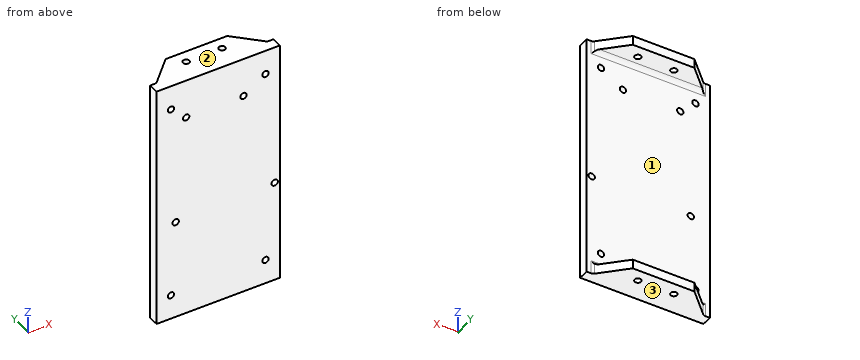
Autodesk Inventor part; units mm, degrees
ref_plane "YZ Plane" through (0, 0, 0) normal (1, 0, 0) x (0, 1, 0)
ref_plane "XZ Plane" through (0, 0, 0) normal (0, 1, 0) x (-1, 0, 0)
ref_plane "XY Plane" through (0, 0, 0) normal (0, 0, 1) x (1, 0, 0)
sketch "Sketch1" plane through (0, 0, 0) normal (0, 1, 0) x (-1, 0, 0)
  line L0 (0, 0) -> (60, 0)
  line L1 (60, 0) -> (60, -120)
  line L2 (60, -120) -> (0, -120)
  line L3 (0, -120) -> (0, 0)
  dimension "d0" = 60
  dimension "d1" = 120
extrude "Extrusion1" add sketch "Sketch1" along normal blind 5
sketch "Sketch2" plane through (0, 5, 0) normal (0, 1, 0) x (1, 0, 0)
  line L0 (-30, 120) -> (-45, 120)
  line L1 (-30, 120) -> (-15, 120)
  line L2 (-45, 120) -> (-45, 115.5)
  line L3 (-45, 115.5) -> (-15, 115.5)
  line L4 (-15, 115.5) -> (-15, 120)
  line L5 (-15, 120) -> (-45, 120)
  line L6 (-60, 120) -> (-60, 0)
  line L7 (0, 0) -> (0, 120)
  line L8 (-30, 0) -> (-45, 0)
  line L9 (-30, 0) -> (-15, 0)
  line L10 (-45, 0) -> (-45, 4.5)
  line L11 (-45, 4.5) -> (-15, 4.5)
  line L12 (-15, 4.5) -> (-15, 0)
  line L13 (-45, 0) -> (-15, 0)
  line L14 (-60, 0) -> (0, 0)
  dimension "d9" = 15
  dimension "d10" = 15
  dimension "d12" = 4.5
extrude "Extrusion2" add sketch "Sketch2" along normal blind 12
chamfer "Chamfer1" distance 12 angle 45 4 edges at (-45, 5, -2.25) (-45, 5, -117.75) (-15, 5, -2.25) (-15, 5, -117.75)
fillet "Fillet1" radius 2 6 edges at (-30, 5, -115.5) (-56.9995, 5, -117.75) (-56.9995, 5, -2.25) (-30, 5, -4.5) (-3.0005, 5, -2.25) (-3.0005, 5, -117.75)
sketch "Sketch3" plane through (-60, 0, 0) normal (0, 0, 1) x (1, 0, 0)
  line L0 (0, 0) -> (60, 0)
  circle A0 centre (38.75, 11) radius 1.55
  circle A1 centre (21.25, 11) radius 1.55
  dimension "d22" = 3.1
  dimension "d23" = 3.1
  dimension "d25" = 17.5
  dimension "d26" = 11
  dimension "d27" = 11
extrude "Extrusion3" cut sketch "Sketch3" against normal through all
sketch "Sketch4" plane through (0, 5, 0) normal (0, 1, 0) x (1, 0, 0)
  line L0 (0, 0) -> (0, 120)
  line L1 (0, 50.8517) -> (-60, 50.8517)
  line L2 (-60, 120) -> (-60, 0)
  line L3 (-26.65, 16.5517) -> (0, 16.5517)
  line L4 (0, 16.5517) -> (0, 85.1517)
  line L5 (0, 85.1517) -> (-53.3, 85.1517)
  line L6 (-53.3, 85.1517) -> (-53.3, 16.5517)
  line L7 (-53.3, 16.5517) -> (-26.65, 16.5517)
  line L8 (0, 85.1517) -> (0, 84.5517)
  line L9 (0, 85.1517) -> (0, 69.8517)
  circle A0 centre (-2.5, 69.8517) radius 1.55
  line L10 (-26.65, 85.1517) -> (-26.65, 16.5517)
  circle A1 centre (-50.7, 71.1517) radius 1.55
  circle A2 centre (-17.7, 19.0517) radius 1.55
  circle A3 centre (-45.6, 19.0517) radius 1.55
  line L11 (0, 85.1517) -> (-2, 85.1517)
  dimension "d34" = 53.3
  dimension "d35" = 68.6
  dimension "d39" = 3.1
  dimension "d43" = 3.1
  dimension "d44" = 3.1
  dimension "d55" = 14
  dimension "d56" = 1.3
  dimension "d57" = 50.8
  dimension "d58" = 15.2
  dimension "d59" = 27.9
extrude "Extrusion4" cut sketch "Sketch4" against normal blind 12 contours A0 | A1 | A2 | A3
sketch "Sketch5" plane through (0, 5, 0) normal (0, 1, 0) x (1, 0, 0)
  line L0 (0, 0) -> (0, 120)
  line L1 (0, 120) -> (0, 108)
  line L2 (0, 108) -> (-7, 108)
  line L3 (-60, 120) -> (-60, 0)
  circle A0 centre (-7, 108) radius 1.55
  line L4 (0, 120) -> (-60, 120)
  line L5 (-30, 120) -> (-30, 0)
  line L6 (-45, 0) -> (-15, 0)
  line L7 (0, 60) -> (-60, 60)
  circle A1 centre (-53, 108) radius 1.55
  circle A2 centre (-7, 12) radius 1.55
  circle A3 centre (-53, 12) radius 1.55
  dimension "d47" = 12
  dimension "d48" = 7
  dimension "d49" = 3.1
extrude "Extrusion5" cut sketch "Sketch5" against normal blind 10 contours A0 | A1 | A2 | A3
properties part number "bottom_plate" material "PET Plastic"
Source: CAD feature listing. Evaluate the final solid. Frame: model axes, mm. Face numbers are marked on the shaded views. Round coordinates to 2 decimals unless told otherwise and drop trailing zeros. Write each loop counter-clockwise with the first axis right and the second up, starting at its lowest first coordinate (ties: lowest second). Pieces come first, ordered by that corner, then holes. Notation, with made-up numbers: M 56,77 L 94,77 A28 cw 94,108 Z; hole C -25.75,72 d4. An arc over 180 degrees is marked long. Use CSV: the item, a comma, the result in double quotes. Start each with the question number.
Q1. Pull-direction query (Z, two-part tool) for the marked faces 1, 2 and 3; classes: +Z half, -Z half, draft (parallel to the pull), parting line (faces both ways), or undercut.
Q2. Cut plane A-A on z = -108. Output: boundary loops of the cut face in (x, y).
Q3. Cut plane D-D on x = -12. Output: boundary loops of the cut face in (y, z), plus the area to 3 significant figures.
Q4. Line query: line 1 (X direction, y = 1.3, z = -108); line 2 (Z direction, x = -42, y = 10); line 3 (Y direction, x = -21.25, z = -1.7). Output: solid intervals per line, ascending. Write a range as from..to.
Q5. First-contact query: P1, Ø6, axis at x = -9.5, z = -28.5, coming from the +Y side; P2, Ø2.5, axis at x = -38.75, y = 11, coming from the -Z side. Flat tips, straight axial feed; report the tip coordinate or a pass-through.
Q6. Cut plane B-B on x = -38.75. Output: boundary loops of the cut face in (y, z).
Q7. Cut plane C-C on y = 11. Output: boundary loops of the cut face in (x, z).
Results found:
1,face 1,"undercut"
1,face 2,"+Z half"
1,face 3,"-Z half"
2,outline,"M -60,0 L -54.55,0 L -54.55,5 L -60,5 Z; M -51.45,0 L -8.55,0 L -8.55,5 L -51.45,5 Z; M -5.45,0 L 0,0 L 0,5 L -5.45,5 Z"
3,outline,"M 0,-120 L 14,-120 L 14,-115.5 L 7,-115.5 A2 cw 5,-113.5 L 5,-6.5 A2 cw 7,-4.5 L 14,-4.5 L 14,0 L 0,0 Z"
3,area,"683 mm^2"
4,line 1,"-60..-54.55, -51.45..-8.55, -5.45..0"
4,line 2,"-120..-115.5, -4.5..0"
4,line 3,"0..9.45, 12.55..17"
5,P1,"y = 5"
5,P2,"through"
6,outline,"M 0,-120 L 9.45,-120 L 9.45,-115.5 L 7,-115.5 A2 cw 5,-113.5 L 5,-6.5 A2 cw 7,-4.5 L 9.45,-4.5 L 9.45,0 L 0,0 Z; M 12.55,-120 L 17,-120 L 17,-115.5 L 12.55,-115.5 Z; M 12.55,-4.5 L 17,-4.5 L 17,0 L 12.55,0 Z"
7,outline,"M -51,-120 L -40.3,-120 L -40.3,-115.5 L -51,-115.5 Z; M -51,-4.5 L -40.3,-4.5 L -40.3,0 L -51,0 Z; M -37.2,-120 L -22.8,-120 L -22.8,-115.5 L -37.2,-115.5 Z; M -37.2,-4.5 L -22.8,-4.5 L -22.8,0 L -37.2,0 Z; M -19.7,-120 L -9,-120 L -9,-115.5 L -19.7,-115.5 Z; M -19.7,-4.5 L -9,-4.5 L -9,0 L -19.7,0 Z"
